```python
from build123d import *

# Parameters (mm, degrees)
SKETCH1_W           = 19
SKETCH1_H           = 19
BOSS_EXTRUDE1_DEPTH = 11
SKETCH2_R           = 7.5
BOSS_EXTRUDE2_DEPTH = 8
SKETCH4_R           = 8.5
BOSS_EXTRUDE3_DEPTH = 4
SKETCH3_R           = 1
CUT_EXTRUDE1_DEPTH  = 36.369478368


with BuildPart() as part:
    # Sketch1 → Boss-Extrude1 (new body)
    with BuildSketch(Plane.XY):
        with Locations((9.5, 9.5)):
            Rectangle(SKETCH1_W, SKETCH1_H)
    extrude(amount=BOSS_EXTRUDE1_DEPTH)

    # Sketch2 → Boss-Extrude2 (add)
    with BuildSketch(Plane.XY.offset(11)):
        with Locations(Location((9.5, 9.5, 0), (0, 0, 180))):
            Circle(SKETCH2_R)
    extrude(amount=BOSS_EXTRUDE2_DEPTH)

    # Sketch4 → Boss-Extrude3 (add)
    with BuildSketch(Plane.XY.offset(19)):
        with Locations((9.5, 9.5)):
            Circle(SKETCH4_R)
    extrude(amount=BOSS_EXTRUDE3_DEPTH)

    # Sketch3 → Cut-Extrude1 (cut, through all)
    with BuildSketch(Plane(origin=(19, 0, 0), x_dir=(0, 0, -1), z_dir=(1, 0, 0))):
        with Locations((-9, 9.5)):
            Circle(SKETCH3_R)
    extrude(amount=-CUT_EXTRUDE1_DEPTH, mode=Mode.SUBTRACT)


solid = part.part
```
Here's how the part is built. I have some questions about the finished solid (model axes, mm). A direction names the side the tool comes from. Give positions to 0.01 mm unless a question says otherwise; leave off trailing zeros. Loops run counter-clockwise (first coordinate to the right, second up) from the corner with the lowest first, then second, coordinate; pieces in that order, holes last. Notation, with made-up numbers: (-29, -18.5) -> (21, -18.5) arc R18 cw to (21, -8.5) -> close; hole circle Ø10 at (34.25, 62.5). An arc over 180 degrees is marked (long way). Use one line per item in the form item = value. Start each with the question number.
1) Which directions (+Z, -Z, +X, -X, +Y, -Y) give clear straight access to the entire face, cutting with the end or side of a thin tool? Please do faces 1 (the face through (11.13, 16.82, 14.94)), 2 (the face through (2.755, 4.328, 20.972)), 3 (the face through (9.63, 10.49, 9.13)).
2) Thinking about a two-plate mould opening in Z: for faces 4 (the face through (9, 10, 23)), 5 (the face through (3, 14, 11)), 6 (the face through (19, 9, 5)), which applies, +Z half, -Z half, draft (parallel to the pull), parting line (faces both ways), or undercut?
3) Imagine slicing it at B-B (z = 9). Please give me the cut outline in (x, y).
4) Imagine slicing it at C-C (x = 9.5). Please give me the cut outline in (y, z).
5) For P1, Ø5, axis at x = 10, z = 19, coming from the +Y side; P2, Ø6, axis at y = 11.5, z = 4, coming from the -X side; P3, Ø8, axis at y = 16.5, z = 16, coming from the -X side; P4, Ø8, axis at x = 13, z = 16, coming from the -Y side, each with a flat end and sliding along its axis, tell me the tip position at first contact or that it passes through.
6) Please list where these lines run through material, in increasing order: line 1 along Z through (x, y) = (1.5, 7.5); line 2 along Y through (x, z) = (3.25, 9.25); line 3 along Z through (x, y) = (16, 17.75).
7) Imagine slicing it at A-A (y = 9.5). Please give me the cut outline in (x, z), then the cut area to 3 significant figures.
8) Imagine slicing it at D-D (z = 19.5). Please give me the cut outline in (x, y).
Check values:
q1.face_1 = none
q1.face_2 = +Z
q1.face_3 = +X, -X
q2.face_4 = +Z half
q2.face_5 = undercut
q2.face_6 = draft
q3.outline = (0, 0) -> (19, 0) -> (19, 8.5) -> (0, 8.5) -> close; (0, 10.5) -> (19, 10.5) -> (19, 19) -> (0, 19) -> close
q4.outline = (0, 0) -> (19, 0) -> (19, 11) -> (17, 11) -> (17, 19) -> (18, 19) -> (18, 23) -> (1, 23) -> (1, 19) -> (2, 19) -> (2, 11) -> (0, 11) -> close; hole circle Ø2 at (9.5, 9)
q5.P1 = 18
q5.P2 = 0
q5.P3 = 2.2
q5.P4 = 1.04
q6.line_1 = 0 to 11, 19 to 23
q6.line_2 = 0 to 8.53, 10.47 to 19
q6.line_3 = 0 to 11
q7.outline = (0, 0) -> (19, 0) -> (19, 8) -> (0, 8) -> close; (0, 10) -> (19, 10) -> (19, 11) -> (17, 11) -> (17, 19) -> (18, 19) -> (18, 23) -> (1, 23) -> (1, 19) -> (2, 19) -> (2, 11) -> (0, 11) -> close
q7.area = 359 mm^2
q8.outline = circle Ø17 at (9.5, 9.5)
